Design review of the part built by this model. Coordinates are the model's own, in mm. A direction names the side the tool comes from. Coordinates: 2 decimals unless noted, no trailing zeros. Loops run counter-clockwise (first coordinate to the right, second up) from the corner with the lowest first, then second, coordinate; pieces in that order, holes last. Notation, with made-up numbers: M 3,-38 L 25,-38 A20 ccw 25,-15 Z; hole C 7,-29.5 d11. An arc over 180 degrees is marked long. Answer as a JSON object with one key per item and string values. Group by question number.
1. Consider section B-B (x = 8). State the section outline as (y, z) points, then the cut area to 3 significant figures.
2. Machinability: for faces 1 (the cylindrical face through (11.43, -1.5, 12.02)), 2 (the flat face through (-5, -2, 0)), 3 (the flat face through (-5, -2, 14.5)), 4 (the flat face through (15.5, 0, 7)), 5 (the flat face through (-7.25, 2, 2)), which of the approach directions +Z, -Z, +X, -X, +Y, -Y give a long, thin tool a straight path to every point of the face, cutting with its end or side? Answer none if there is none.
3. Consider section A-A (y = 0). State the section outline as (x, z) points, then the cut area to 3 significant figures.
4. Consider section C-C (z = 20.5). State the section outline as (x, y) points.
5. To check wall thickness, follow probe 1 along X at (y, z) = (-5.25, 7); probe 2 along Z at (x, y) = (6, -3.5); probe 3 along Y at (x, z) = (9.5, 11.5). State the ranges of each line that lie inside material, in increasing order.
6. Insertion check: pin 1 (2 mm diameter, centred on x = -12.5, z = 1, fed in from -Y); pin 2 (10 mm diameter, centred on x = 10.5, z = 1.5, fed in from -Y). Each pin has a flat end and moves straight along its axis. Give the tip position at first contact, or say it passes through.
from build123d import *

# Parameters (mm, degrees)
SKETCH1_W           = 14.5
SKETCH1_H           = 14.5
BOSS_EXTRUDE1_DEPTH = 14.5
SKETCH6_R           = 5
BOSS_EXTRUDE2_DEPTH = 15.5
SKETCH7_R           = 5
BOSS_EXTRUDE3_DEPTH = 15.5


with BuildPart() as part:
    # Sketch1 → Boss-Extrude1 (new body)
    with BuildSketch(Plane.XY):
        Rectangle(SKETCH1_W, SKETCH1_H)
    extrude(amount=BOSS_EXTRUDE1_DEPTH)

    # Sketch5 → Cut-Revolve1 (revolve, cut)
    with BuildSketch(Plane(origin=(3.625, 0, 3.625), x_dir=(-0.7071067811865477, 0, 0.7071067811865475), z_dir=(-0.7071067811865475, 0, -0.7071067811865477))):
        with BuildLine():
            Line((12.376524164, 7.25), (16.846797481, 7.25))
            Line((16.846797481, 7.25), (16.846797481, -7.25))
            Line((16.846797481, -7.25), (12.376524164, -7.25))
            ThreePointArc((12.376524164, -7.25), (15.489035507, 0), (12.376524164, 7.25))
        make_face()
    revolve(axis=Axis((0, 7.25, 7.25), (0, -1, 0)), mode=Mode.SUBTRACT)

    # Sketch6 → Boss-Extrude2 (add, symmetric)
    with BuildSketch(Plane(origin=(0, 0, 0), x_dir=(0, 0, -1), z_dir=(1, 0, 0))):
        with Locations(Location((-7.25, 0, 0), (0, 0, 180))):
            Circle(SKETCH6_R)
    extrude(amount=BOSS_EXTRUDE2_DEPTH, both=True)

    # Sketch7 → Boss-Extrude3 (add, symmetric)
    with BuildSketch(Plane(origin=(0, 0, 7.25), x_dir=(-1, 0, 0), z_dir=(0, 0, -1))):
        Circle(SKETCH7_R)
    extrude(amount=BOSS_EXTRUDE3_DEPTH, both=True)


solid = part.part
Findings below:
{
 "1": {"outline": "C 0,7.25 d10", "area": "78.5 mm^2"},
 "2": {"face 1": "+X", "face 2": "-Z", "face 3": "+Z", "face 4": "+Z, -Z, +X, +Y, -Y", "face 5": "-X"},
 "3": {"outline": "M -15.5,2.25 L -7.25,2.25 L -7.25,0 L -5,0 L -5,-8.25 L 5,-8.25 L 5,0 L 7.25,0 L 7.25,2.25 L 15.5,2.25 L 15.5,12.25 L 7.25,12.25 L 7.25,14.5 L 5,14.5 L 5,22.75 L -5,22.75 L -5,14.5 L -7.25,14.5 L -7.25,12.25 L -15.5,12.25 Z", "area": "540 mm^2"},
 "4": {"outline": "C 0,0 d10"},
 "5": {"probe 1": "x = -7.25 to 7.25", "probe 2": "z = 0 to 14.5", "probe 3": "y = -2.63 to 2.63"},
 "6": {"pin 1": "passes through", "pin 2": "stops at y = -7.25"}
}
